Part model, mm, in its own coordinate system. A direction names the side the tool comes from. Give positions to 0.01 mm unless a question says otherwise; leave off trailing zeros. Write each loop counter-clockwise with the first axis right and the second up, starting at its lowest first coordinate (ties: lowest second). Pieces come first, ordered by that corner, then holes. Notation, with made-up numbers: M 11,64 L 60,64 A13 ccw 60,79 Z; hole C 57,-32 d1. An arc over 180 degrees is marked long. Use CSV: the item, a comma, the result in double quotes. Start each with the question number.
1. Drill centre lines: line 1 along Z through (x, y) = (3.25, 3.5); line 2 along Z through (x, y) = (0.75, -1); line 3 along Y through (x, z) = (-1.75, -1) (3 decimals). Where is each one in solid material? Low to high. Write a range as from..to.
2. Drop flat-ended pins along their axis: pin 1 Ø0.7 at (x, z) = (4.5, 5.5) entering from -Y; pin 2 Ø0.8 at (x, z) = (-4, 5.5) entering from +Y; pin 3 Ø4 at (y, z) = (2.5, -2.5) entering from -X (3 decimals). Give the stop position or say it passes through.
3. Band-saw the part on A-A, the plane z = -0.5. List the corners of the cut face in (x, y) (3 decimals).
4. Band-saw the part on C-C, the plane y = -2.5. List the corners of the cut face in (x, z), then the cut area to 3 significant figures.
5. 3-axis set-ups, long thin cutter, end or side, ignore diameter. For faces 1 (the face through (1, 0.675, -2)), 2 (the face through (-1.5, 1.424, 5.4)), 3 (the face through (-3.5, -1.626, 5.4)), 4 (the face through (-3.798, 0.2, 5.4)): which of +Z, -Z, +X, -X, +Y, -Y reach the whole face in a straight line?
6. Mould opens along X. For faces 5 (the face through (0, 2.025, -2)), 6 (the face through (-0.75, -5.7, 2.46)), 7 (the face through (3.871, -0.4, 5.4)) say: pulls with the +X half, pulls with the -X half, needs draft (parallel to the pull), parting line crosses it, or undercut.
7. Band-saw the part on B-B, the plane x = -3.5. List the corners of the cut face in (y, z).
8. Band-saw the part on D-D, the plane z = 2.5. List the corners of the cut face in (x, y).
Autodesk Inventor part; units mm, degrees
ref_plane "YZ Plane" through (0, 0, 0) normal (1, 0, 0) x (0, 1, 0)
ref_plane "XZ Plane" through (0, 0, 0) normal (0, 1, 0) x (-1, 0, 0)
ref_plane "XY Plane" through (0, 0, 0) normal (0, 0, 1) x (1, 0, 0)
sketch "Sketch1" plane through (0, 0, 0) normal (0, 0, 1) x (1, 0, 0)
  circle A0 centre (0, 0) radius 6.22 construction
  circle A1 centre (0, 0) radius 2.8
  line L0 (-0.675, 0.675) -> (-0.675, 2.025)
  line L1 (-0.675, 2.025) -> (0.675, 2.025)
  line L2 (0.675, 2.025) -> (0.675, 0.675)
  line L3 (0.675, 0.675) -> (2.025, 0.675)
  line L4 (2.025, 0.675) -> (2.025, -0.675)
  line L5 (2.025, -0.675) -> (0.675, -0.675)
  line L6 (0.675, -0.675) -> (0.675, -2.025)
  line L7 (0.675, -2.025) -> (-0.675, -2.025)
  line L8 (-0.675, -2.025) -> (-0.675, -0.675)
  line L9 (-0.675, -0.675) -> (-2.025, -0.675)
  line L10 (-2.025, -0.675) -> (-2.025, 0.675)
  line L11 (-2.025, 0.675) -> (-0.675, 0.675)
  circle A2 centre (0, 0) radius 5.75
  point P0 (-6.07, -6.1)
  dimension "d0" = 12.44
  dimension "d1" = 0.47
extrude "Extrusion1" add sketch "Sketch1" along normal blind 5 contours A1 | L0 L1 L2 L3 L4 L5 L6 L7 L8 L9 L10 L11 | A2
extrude "Extrusion2" add sketch "Sketch1" against normal blind 4.8 contours A1
sketch "Sketch2" plane through (0, 0, 5) normal (0, 0, 1) x (1, 0, 0)
  point P0 (0, 0)
sketch "Sketch3" plane through (0, 0, 5) normal (0, 0, 1) x (1, 0, 0)
  line L0 (-4.8809, 1.4783) -> (4.8809, 1.4783) construction
  line L1 (4.8809, 1.4783) -> (4.8809, -1.6654) construction
  line L2 (4.8809, -1.6654) -> (-4.8809, -1.6654) construction
  line L3 (-4.8809, -1.6654) -> (-4.8809, 1.4783) construction
  line L4 (-2.5303, -1.6261) -> (-4.5645, -1.6261)
  line L5 (-4.5645, -1.6261) -> (-4.5645, 1.4239)
  line L6 (-4.5645, 1.4239) -> (-3.7983, 1.4239)
  line L7 (-3.7983, 1.4239) -> (-3.7983, -1.0452)
  line L8 (-3.7983, -1.0452) -> (-2.5303, -1.0452)
  line L9 (-2.5303, -1.0452) -> (-2.5303, -1.6261)
  line L10 (-0.6469, -1.6261) -> (-2.2881, -1.6261)
  line L11 (-2.2881, -1.6261) -> (-2.2881, -1.0947)
  line L12 (-2.2881, -1.0947) -> (-1.8506, -1.0947)
  line L13 (-1.8506, -1.0947) -> (-1.8506, 0.8925)
  line L14 (-1.8506, 0.8925) -> (-2.2881, 0.8925)
  line L15 (-2.2881, 0.8925) -> (-2.2881, 1.4239)
  line L16 (-2.2881, 1.4239) -> (-0.6469, 1.4239)
  line L17 (-0.6469, 1.4239) -> (-0.6469, 0.8925)
  line L18 (-0.6469, 0.8925) -> (-1.0844, 0.8925)
  line L19 (-1.0844, 0.8925) -> (-1.0844, -1.0947)
  line L20 (-1.0844, -1.0947) -> (-0.6469, -1.0947)
  line L21 (-0.6469, -1.0947) -> (-0.6469, -1.6261)
  spline S0 degree 2 poles (0.8039, -1.6804) (0.4529, -1.6804) (-0.076, -1.5445) (-0.3034, -1.4456) knots 0 0 0 1 2 2 2
  line L22 (-0.3034, -1.4456) -> (-0.3034, -0.719)
  line L23 (-0.3034, -0.719) -> (-0.2342, -0.719)
  spline S1 degree 2 poles (-0.2342, -0.719) (-0.0043, -0.9142) (0.5469, -1.1243) (0.8064, -1.1243) knots 0 0 0 1 2 2 2
  spline S2 degree 2 poles (0.8064, -1.1243) (0.8731, -1.1243) (1.0882, -1.0947) (1.1524, -1.065) knots 0 0 0 1 2 2 2
  spline S3 degree 2 poles (1.1524, -1.065) (1.2315, -1.0304) (1.3427, -0.9044) (1.3427, -0.803) knots 0 0 0 1 2 2 2
  spline S4 degree 2 poles (1.3427, -0.803) (1.3427, -0.6868) (1.1623, -0.5435) (1.0387, -0.5114) knots 0 0 0 1 2 2 2
  spline S5 degree 2 poles (1.0387, -0.5114) (0.883, -0.4693) (0.5296, -0.3977) (0.3738, -0.3433) knots 0 0 0 1 2 2 2
  spline S6 degree 2 poles (0.3738, -0.3433) (0.0204, -0.2197) (-0.2861, 0.2029) (-0.2861, 0.5193) knots 0 0 0 1 2 2 2
  spline S7 degree 2 poles (-0.2861, 0.5193) (-0.2861, 0.9469) (0.4381, 1.4783) (0.9819, 1.4783) knots 0 0 0 1 2 2 2
  spline S8 degree 2 poles (0.9819, 1.4783) (1.2538, 1.4783) (1.7926, 1.3671) (2.0051, 1.2732) knots 0 0 0 1 2 2 2
  line L24 (2.0051, 1.2732) -> (2.0051, 0.5762)
  line L25 (2.0051, 0.5762) -> (1.9384, 0.5762)
  spline S9 degree 2 poles (1.9384, 0.5762) (1.7679, 0.722) (1.2785, 0.9222) (1.0214, 0.9222) knots 0 0 0 1 2 2 2
  spline S10 degree 2 poles (1.0214, 0.9222) (0.9201, 0.9222) (0.7619, 0.8925) (0.6729, 0.853) knots 0 0 0 1 2 2 2
  spline S11 degree 2 poles (0.6729, 0.853) (0.6012, 0.8209) (0.4974, 0.6923) (0.4974, 0.6132) knots 0 0 0 1 2 2 2
  spline S12 degree 2 poles (0.4974, 0.6132) (0.4974, 0.4946) (0.663, 0.3587) (0.9003, 0.3043) knots 0 0 0 1 2 2 2
  spline S13 degree 2 poles (0.9003, 0.3043) (1.0535, 0.2697) (1.3378, 0.2029) (1.5009, 0.1461) knots 0 0 0 1 2 2 2
  spline S14 degree 2 poles (1.5009, 0.1461) (1.8173, 0.0299) (2.1262, -0.3556) (2.1262, -0.672) knots 0 0 0 1 2 2 2
  spline S15 degree 2 poles (2.1262, -0.672) (2.1262, -1.1268) (1.4119, -1.6804) (0.8039, -1.6804) knots 0 0 0 1 2 2 2
  line L26 (3.105, -1.6261) -> (3.105, 0.8431)
  line L27 (3.105, 0.8431) -> (2.2029, 0.8431)
  line L28 (2.2029, 0.8431) -> (2.2029, 1.4239)
  line L29 (2.2029, 1.4239) -> (4.7734, 1.4239)
  line L30 (4.7734, 1.4239) -> (4.7734, 0.8431)
  line L31 (4.7734, 0.8431) -> (3.8712, 0.8431)
  line L32 (3.8712, 0.8431) -> (3.8712, -1.6261)
  line L33 (3.8712, -1.6261) -> (3.105, -1.6261)
  point P0 (0, -1.6654)
  point P1 (0, 0)
  point P2 (0, 0)
extrude "Extrusion5" add sketch "Sketch3" along normal blind 0.9
properties part number "IPC List key"
Output:
1,line 1,"z = 0..5"
1,line 2,"z = -4.8..5"
1,line 3,"y = -2.186..-0.675, 0.675..2.186"
2,pin 1,"stops at y = 0.84"
2,pin 2,"stops at y = 1.42"
2,pin 3,"stops at x = -2.755"
3,outline,"C 0,0 d5.6; hole M -2.025,-0.675 L -0.675,-0.675 L -0.675,-2.025 L 0.675,-2.025 L 0.675,-0.675 L 2.025,-0.675 L 2.025,0.675 L 0.675,0.675 L 0.675,2.025 L -0.675,2.025 L -0.675,0.675 L -2.025,0.675 Z"
4,outline,"M -5.18,0 L -1.26,0 L -1.26,-4.8 L 1.26,-4.8 L 1.26,0 L 5.18,0 L 5.18,5 L -5.18,5 Z"
4,area,"63.9 mm²"
5,face 1,"-Z"
5,face 2,"+Z, -X, +Y"
5,face 3,"+Z, -X, -Y"
5,face 4,"+Z, +Y"
6,face 5,"undercut"
6,face 6,"parting line crosses it"
6,face 7,"pulls with the +X half"
7,outline,"M -4.56,0 L 4.56,0 L 4.56,5 L -1.05,5 L -1.05,5.9 L -1.63,5.9 L -1.63,5 L -4.56,5 Z"
8,outline,"C 0,0 d11.5"
